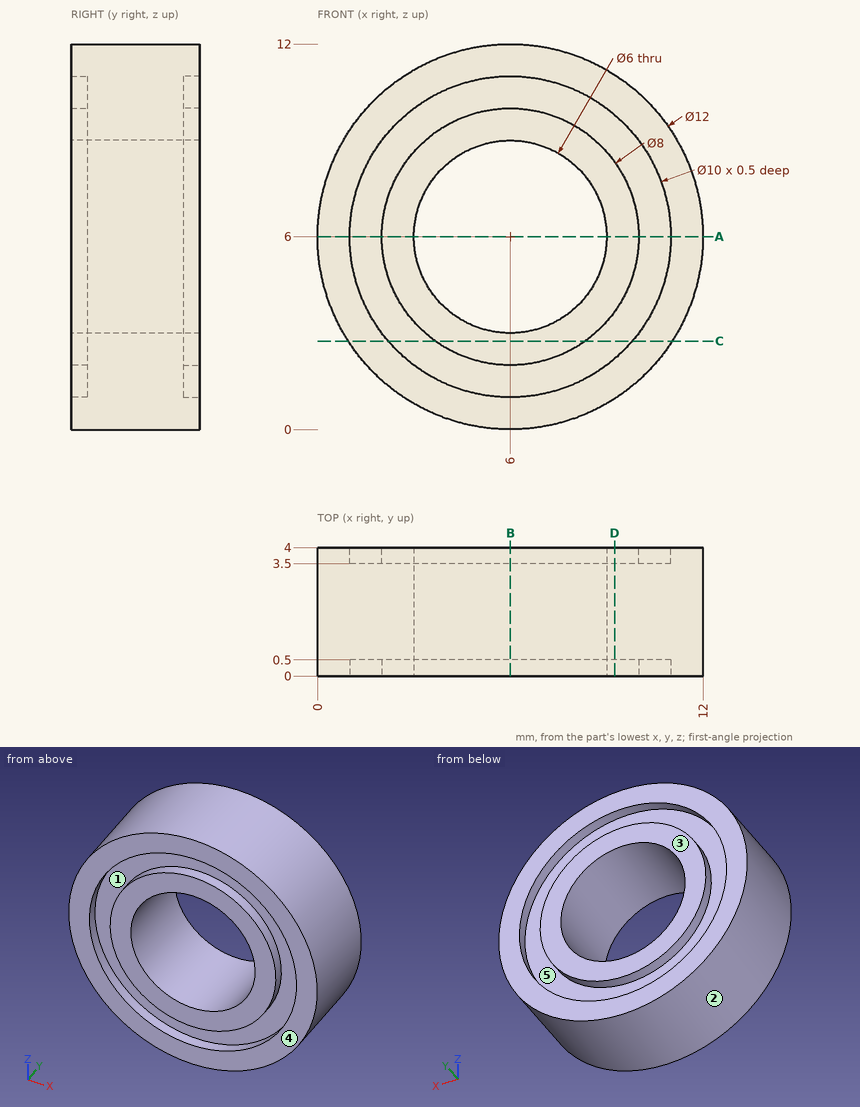
Print and shaded views of the part. All mm, measured from the part's lowest x, y and z. A direction names the side the tool comes from. Round coordinates to 2 decimals unless told otherwise and drop trailing zeros. Write each loop counter-clockwise with the first axis right and the second up, starting at its lowest first coordinate (ties: lowest second). Pieces come first, ordered by that corner, then holes.
Item 1: Cut at B-B, the plane x = 6. Give the cut face in (y, z), plus the area to 3 significant figures.
Results:
outline: (0, 0) - (4, 0) - (4, 1) - (3.5, 1) - (3.5, 2) - (4, 2) - (4, 3) - (0, 3) - (0, 2) - (0.5, 2) - (0.5, 1) - (0, 1) - close; (0, 9) - (4, 9) - (4, 10) - (3.5, 10) - (3.5, 11) - (4, 11) - (4, 12) - (0, 12) - (0, 11) - (0.5, 11) - (0.5, 10) - (0, 10) - close
area: 22.0 mm2
Item 2: Probe L1, parallel to X at y = 0.2, z = 6; L2, parallel to X at y = 2.25, z = 6; L3, parallel to X at y = 3.1, z = 4.5. List the from-to ranges inside material, lowest first.
Results:
L1: x = 0 to 1, 2 to 3, 9 to 10, 11 to 12
L2: x = 0 to 3, 9 to 12
L3: x = 0.19 to 3.4, 8.6 to 11.81
Item 3: Cut at C-C, the plane z = 2.75. Give the cut face in (x, y).
Results:
outline: (0.96, 0) - (2.2, 0) - (2.2, 0.5) - (3.67, 0.5) - (3.67, 0) - (8.33, 0) - (8.33, 0.5) - (9.8, 0.5) - (9.8, 0) - (11.04, 0) - (11.04, 4) - (9.8, 4) - (9.8, 3.5) - (8.33, 3.5) - (8.33, 4) - (3.67, 4) - (3.67, 3.5) - (2.2, 3.5) - (2.2, 4) - (0.96, 4) - close
Item 4: Cut at A-A, the plane z = 6. Give the cut face in (x, y).
Results:
outline: (0, 0) - (1, 0) - (1, 0.5) - (2, 0.5) - (2, 0) - (3, 0) - (3, 4) - (2, 4) - (2, 3.5) - (1, 3.5) - (1, 4) - (0, 4) - close; (9, 0) - (10, 0) - (10, 0.5) - (11, 0.5) - (11, 0) - (12, 0) - (12, 4) - (11, 4) - (11, 3.5) - (10, 3.5) - (10, 4) - (9, 4) - close
Item 5: Which spindle directions (+Z, -Z, +X, -X, +Y, -Y) get a long thin tool onto all of the face, cutting with end or side? Do the marked faces 4 and 5. Say none if no direction does.
Results:
face 4: +Z, -Z, +X, -X, -Y
face 5: +Y
Item 6: Cut at D-D, the plane x = 9.25. Give the cut face in (y, z).
Results:
outline: (0, 0.96) - (4, 0.96) - (4, 2.2) - (3.5, 2.2) - (3.5, 3.67) - (4, 3.67) - (4, 8.33) - (3.5, 8.33) - (3.5, 9.8) - (4, 9.8) - (4, 11.04) - (0, 11.04) - (0, 9.8) - (0.5, 9.8) - (0.5, 8.33) - (0, 8.33) - (0, 3.67) - (0.5, 3.67) - (0.5, 2.2) - (0, 2.2) - close
Item 7: Drop a flat-ended pin along its axis: pin 1 Ø1.5 at (y, z) = (3.5, 1.5) entering from -X. Give the stop position or say it passes through.
Results:
pin 1: stops at x = 1.32
Item 8: Two-plate mould, pull along X, no slides. Class the marked faces 1, 2 and 3: +X half, -X half, draft (parallel to the pull), parting line (faces both ways), or undercut.
Results:
face 1: undercut
face 2: parting line
face 3: draft
